from build123d import *

# Parameters (mm, degrees)
SKETCH1_R           = 6.35
BOSS_EXTRUDE1_DEPTH = 25.4
SKETCH4_W           = 13.081
SKETCH4_H           = 6.731
CUT_EXTRUDE1_DEPTH  = 6.35
FILLET1_R           = 1.5875


with BuildPart() as part:
    # Sketch1 → Boss-Extrude1 (new body)
    with BuildSketch(Plane.XY):
        Circle(SKETCH1_R)
    extrude(amount=BOSS_EXTRUDE1_DEPTH)

    # Sketch4 → Cut-Extrude1 (cut)
    with BuildSketch(Plane(origin=(6.35, 0, 0), x_dir=(0, 0, -1), z_dir=(1, 0, 0))):
        with Locations((-9.2075, 0)):
            Rectangle(SKETCH4_W, SKETCH4_H)
    extrude(amount=-CUT_EXTRUDE1_DEPTH, mode=Mode.SUBTRACT)

    # Fillet1
    fillet1_edges = [part.edges().sort_by_distance(p)[0] for p in [
        (2.692392512, -3.3655, 15.748),
        (2.692392512, 3.3655, 15.748),
        (2.692392512, 3.3655, 2.667),
        (2.692392512, -3.3655, 2.667),
    ]]
    fillet(fillet1_edges, radius=FILLET1_R)


solid = part.part
Work out the finished part from the listing and answer in its coordinate system (mm). A direction names the side the tool comes from. Give positions to 0.01 mm unless a question says otherwise; leave off trailing zeros. Write each loop counter-clockwise with the first axis right and the second up, starting at its lowest first coordinate (ties: lowest second). Pieces come first, ordered by that corner, then holes.
Q1. The part is cut by section C-C on z = 12. Give the vertices of the cut face in (x, y), and give its area (3 significant figures).
Answer:
outline: (0, -3.37) - (0, 3.37) - (5.38, 3.37) arc R6.35 ccw (long way) to (5.38, -3.37) - close
area: 86.0 mm2
Q2. Straight lines are drawn through the part: L1, parallel to Y at x = 0.25, z = 10.25; L2, parallel to Y at x = 3, z = 13.75; L3, parallel to Z at x = 2.5, y = -0.5. For each, find the intervals that lie inside material, in ascending order.
Answer:
L1: y = -6.35 to -3.37, 3.37 to 6.35
L2: y = -5.6 to -3.37, 3.37 to 5.6
L3: z = 0 to 2.67, 15.75 to 25.4
Q3. The part is cut by section A-A on x = 1.25. Give the vertices of the cut face in (y, z) (1 decimal), and give its area (3 significant figures).
Answer:
outline: (-6.2, 0) - (6.2, 0) - (6.2, 25.4) - (-6.2, 25.4) - close; hole (-3.4, 4.3) arc R1.6 ccw to (-1.8, 2.7) - (1.8, 2.7) arc R1.6 ccw to (3.4, 4.3) - (3.4, 14.2) arc R1.6 ccw to (1.8, 15.7) - (-1.8, 15.7) arc R1.6 ccw to (-3.4, 14.2) - close
area: 230 mm2
Q4. A tool of negligible diameter and unlimited length cuts with its end or side. For faces 5 (the face through (3.01, 2.89, 3.12)), 6 (the face through (0, 0, 25.4)), from which of +Z, -Z, +X, -X, +Y, -Y can it reach the whole face along a straight path? Write none if from no direction.
Answer:
face 5: +X
face 6: +Z, +X, -X, +Y, -Y
Q5. The part is cut by section D-D on y = -2.5. Give the vertices of the cut face in (x, z), and give its area (3 significant figures).
Answer:
outline: (-5.84, 0) - (5.84, 0) - (5.84, 2.84) - (0, 2.84) - (0, 15.57) - (5.84, 15.57) - (5.84, 25.4) - (-5.84, 25.4) - close
area: 222 mm2
Q6. For a pull along Y with two mould halves and no side action, classify faces 1 (the face through (3, 3.366, 9)), 2 (the face through (0, 0, 9)), 3 (the face through (0, 0, 0)), 4 (the face through (-6.344, 0.279, 12.522)) as released by +Y, released by -Y, zero draft, split by the parting line, or undercut.
Answer:
face 1: undercut
face 2: undercut
face 3: zero draft
face 4: split by the parting line
Q7. The part is cut by section B-B on y = 0. Give the vertices of the cut face in (x, z), and give its area (3 significant figures).
Answer:
outline: (-6.35, 0) - (6.35, 0) - (6.35, 2.67) - (0, 2.67) - (0, 15.75) - (6.35, 15.75) - (6.35, 25.4) - (-6.35, 25.4) - close
area: 240 mm2
Q8. Given pin 1 (2.5 mm diameter, centred on x = 4, z = 11, fed in from +Y); pin 2 (3.5 mm diameter, centred on y = 0, z = 9.5, fed in from +X); pin 3 (2 mm diameter, centred on x = 4, z = 7.5, fed in from +Y), each flat-ended and moving along its own axis, determine where each tip first touches the part or whether it passes through.
Answer:
pin 1: stops at y = 5.72
pin 2: stops at x = 0
pin 3: stops at y = 5.6
